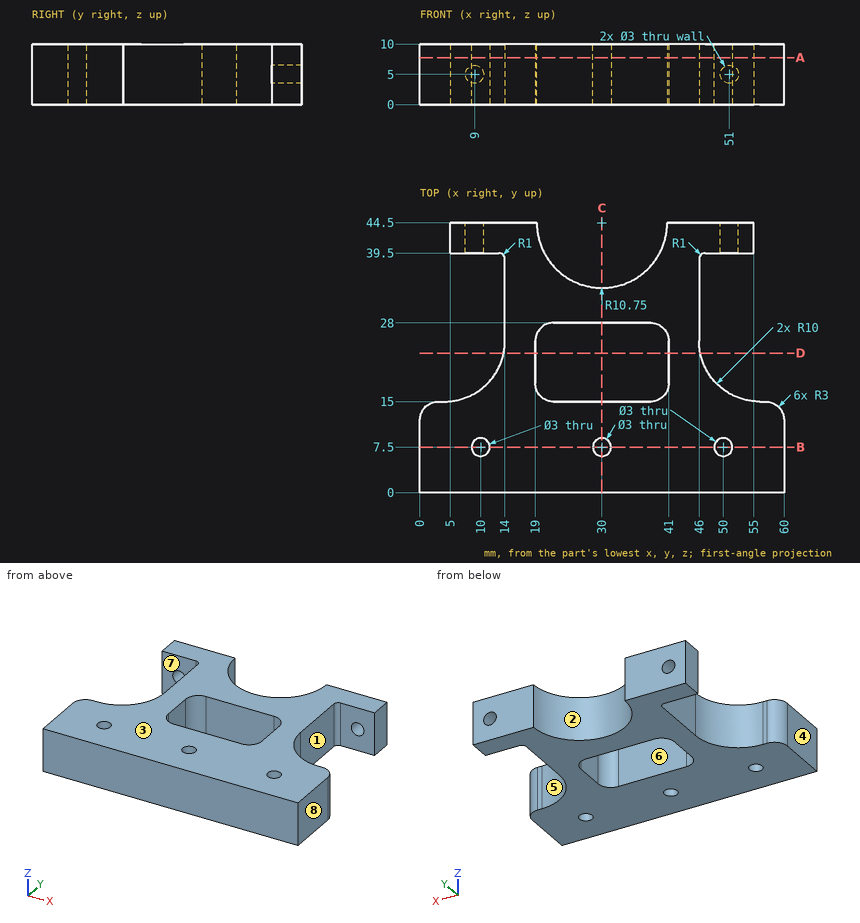
Input: dimensioned drawing with shaded views. Units: mm. Origin: part minimum x, y, z. A direction names the side the tool comes from. Coordinates: 2 decimals unless noted, no trailing zeros. Loops run counter-clockwise (first coordinate to the right, second up) from the corner with the lowest first, then second, coordinate; pieces in that order, holes last. Notation, with made-up numbers: (73.25, -3.5) -> (130.25, -3.5) arc R14 cw to (130.25, 11.5) -> close; hole circle Ø7 at (43, 68). An arc over 180 degrees is marked (long way). One line per item, written item: value. Start each with the question number.
Q1. Mould query, pull axis X, two halves, no side actions, for the marked faces 1, 2 and 3. Classes: pulls with the +X half, pulls with the -X half, needs draft (parallel to the pull), parting line crosses it, or undercut.
Q2. Set-up query: the marked faces 4, 5, 6, 7 and 8. Return all of +Z, -Z, +X, -X, +Y, -Y with unobstructed straight access to the full face (end or side cutting, diameter ignored); none if empty.
Q3. Section query B-B, the plane y = 7.5. Return the cut outline in (x, z), and give its area (3 significant figures).
Q4. Section query A-A, the plane z = 7.75. Give the number of separate pieces and of enclosed holes in the cut face, and give its area (3 significant figures).
Q5. Section query C-C, the plane x = 30. Return the cut outline in (y, z), and give its area (4 significant figures).
Q6. Line query: line 1 along Y through (x, z) = (30, 6.25); line 2 along Y through (x, z) = (50, 7.5); line 3 along X through (y, z) = (40.5, 5). Output: solid intervals per line, ascending.
Q7. Section query D-D, the plane y = 23. Return the cut outline in (x, z).
Q8. Contact query for flat-ended pins moving along their axis: P1, Ø2.5, axis at x = 50, y = 7.5, coming from the -Z side; P2, Ø3, axis at x = 51.5, z = 8.5, coming from the -Y side; P3, Ø5, axis at y = 30, z = 4.5, coming from the -X side; P4, Ø0.8, axis at x = 56.5, z = 3, coming from the +Y side. Output: stop coordinate, or through.
Results:
1. face 1: pulls with the +X half
1. face 2: undercut
1. face 3: needs draft
2. face 4: +Z, -Z, -X, +Y, -Y
2. face 5: +Z, -Z, +X
2. face 6: +Z, -Z
2. face 7: +Z, -Z, -X
2. face 8: +Z, -Z, +X, +Y, -Y
3. outline: (0, 0) -> (8.5, 0) -> (8.5, 10) -> (0, 10) -> close; (11.5, 0) -> (28.5, 0) -> (28.5, 10) -> (11.5, 10) -> close; (31.5, 0) -> (48.5, 0) -> (48.5, 10) -> (31.5, 10) -> close; (51.5, 0) -> (60, 0) -> (60, 10) -> (51.5, 10) -> close
3. area: 510 mm^2
4. separate pieces: 1
4. enclosed holes: 4
4. area: 1,490 mm^2
5. outline: (0, 0) -> (6, 0) -> (6, 10) -> (0, 10) -> close; (9, 0) -> (15, 0) -> (15, 10) -> (9, 10) -> close; (28, 0) -> (33.75, 0) -> (33.75, 10) -> (28, 10) -> close
5. area: 177.5 mm^2
6. line 1: 0 to 6, 9 to 15, 28 to 33.75
6. line 2: 0 to 6, 9 to 17, 39.5 to 44.5
6. line 3: 5 to 7.5, 10.5 to 20.02, 39.98 to 49.5, 52.5 to 55
7. outline: (13.8, 0) -> (19, 0) -> (19, 10) -> (13.8, 10) -> close; (41, 0) -> (46.2, 0) -> (46.2, 10) -> (41, 10) -> close
8. P1: through
8. P2: y = 0
8. P3: x = 14
8. P4: y = 15
